Model file for the job. Use its own axes, mm. A direction names the side the tool comes from. Round coordinates to 2 decimals unless told otherwise and drop trailing zeros. Order: outer loops, then holes, each group sorted by start corner. A loop starts at its lowest first (then second) coordinate and runs counter-clockwise, first axis right, second up. Notation, with made-up numbers: (41, 84) - (80, 84) arc R35 cw to (80, 118) - close; hole circle Ø9 at (31, 27.25). An arc over 180 degrees is marked (long way). Answer as CSV lines item,"result". Start each with the question number.
1. Wall check: line 1 along Z through (x, y) = (-33, 35); line 2 along Y through (x, z) = (-4.5, 33.5); line 3 along Z through (x, y) = (-7, 17.5). Give the ranges that are in metal, low to high. Write a range as [from, to].
2. Band-saw the part on D-D on x = -34. List the corners of the cut face in (y, z).
3. Pin check, flat tips, straight feed: pin 1 Ø1.5 at (x, y) = (-9, 22) entering from +Z; pin 2 Ø2.5 at (x, y) = (-34.25, 9.37) entering from -Z; pin 3 Ø5 at (x, y) = (-3.71, 9.37) entering from -Z; pin 4 Ø2.5 at (x, y) = (-34.25, 39.9) entering from +Z. Stop position of each tip, or through.
4. 3-axis set-ups, long thin cutter, end or side, ignore diameter. For faces 1 (the face through (-35.465, 25.364, 33.504)), 2 (the face through (-39.981, 25, 17)), 3 (the face through (-34, 40, 5)): which of +Z, -Z, +X, -X, +Y, -Y reach the whole face in a straight line?
5. Pull direction Y, two halves, no side cores. Call faces 4 (the face through (-4, 40, 5)), 5 (the face through (-22, 27, 35.75)), 6 (the face through (-37.45, 43.17, 16.64)): released by +Y, released by -Y, zero draft, split by the parting line, or undercut.
6. Band-saw the part on B-B on x = -12.5. List the corners of the cut face in (y, z), then the cut area to 3 significant figures.
7. Band-saw the part on C-C on y = 37. List the corners of the cut face in (x, z), then the cut area to 3 significant figures.
8. Band-saw the part on A-A on z = 6. List the corners of the cut face in (x, y).
```python
from build123d import *

# Parameters (mm, degrees)
BOSS_EXTRUDE1_DEPTH = 33.75
SKETCH2_R           = 16.5
CUT_EXTRUDE1_DEPTH  = 0.5
SKETCH3_R           = 11
BOSS_EXTRUDE2_DEPTH = 2.5
SKETCH4_R           = 3.5
CUT_EXTRUDE2_DEPTH  = 5
BOSS_EXTRUDE3_DEPTH = 27
SKETCH6_R           = 1.5
CUT_EXTRUDE3_DEPTH  = 5


with BuildPart() as part:
    # Sketch1 → Boss-Extrude1 (new body)
    with BuildSketch(Plane.XY):
        Polygon((-34.980846502, 45.63851346), (-39.980846502, 40.63851346), (-39.980846502, 8.63851346), (-34.980846502, 3.63851346), (-2.980846502, 3.63851346), (2.019153498, 8.63851346), (2.019153498, 40.63851346), (-2.980846502, 45.63851346), align=None)
    extrude(amount=BOSS_EXTRUDE1_DEPTH)

    # Sketch2 → Cut-Extrude1 (cut)
    with BuildSketch(Plane.XY.offset(33.75)):
        with Locations((-18.980846502, 24.63851346)):
            Circle(SKETCH2_R)
    extrude(amount=-CUT_EXTRUDE1_DEPTH, mode=Mode.SUBTRACT)

    # Sketch3 → Boss-Extrude2 (add)
    with BuildSketch(Plane.XY.offset(33.25)):
        with Locations((-18.980846502, 24.63851346)):
            Circle(SKETCH3_R)
    extrude(amount=BOSS_EXTRUDE2_DEPTH)

    # Sketch4 → Cut-Extrude2 (cut)
    with BuildSketch(Plane.XY.offset(35.75)):
        with Locations((-18.980846502, 24.63851346)):
            Circle(SKETCH4_R)
    extrude(amount=-CUT_EXTRUDE2_DEPTH, mode=Mode.SUBTRACT)

    # Sketch5 → Boss-Extrude3 (add)
    with BuildSketch(Plane.XY.offset(30.75)):
        with BuildLine():
            Line((-20.480846502, 26.63851346), (-17.480846502, 26.63851346))
            ThreePointArc((-17.480846502, 26.63851346), (-18.980846502, 22.13851346), (-20.480846502, 26.63851346))
        make_face()
    extrude(amount=BOSS_EXTRUDE3_DEPTH)

    # Sketch6 → Cut-Extrude3 (cut)
    with BuildSketch(Plane.XY.offset(33.75)):
        with Locations((-34.247281908, 39.904948866)):
            Circle(SKETCH6_R)
        with Locations((-3.714411096, 39.904948866)):
            Circle(SKETCH6_R)
        with Locations((-3.714411096, 9.372078054)):
            Circle(SKETCH6_R)
        with Locations((-34.247281908, 9.372078054)):
            Circle(SKETCH6_R)
    cut_extrude3 = extrude(amount=-CUT_EXTRUDE3_DEPTH, mode=Mode.SUBTRACT)

    # Mirror1: Cut-Extrude3 across plane
    add(cut_extrude3.mirror(Plane(origin=(0, 0, 16.875), x_dir=(1, 0, 0), z_dir=(0, 0, -1))), mode=Mode.SUBTRACT)


solid = part.part
```
Reply:
1,line 1,"z = [0, 33.75]"
1,line 2,"y = [3.64, 8.09], [10.65, 16.73], [32.55, 38.63], [41.18, 45.64]"
1,line 3,"z = [0, 33.25]"
2,outline,"(3.64, 0) - (7.89, 0) - (7.89, 5) - (10.85, 5) - (10.85, 0) - (38.43, 0) - (38.43, 5) - (41.38, 5) - (41.38, 0) - (45.64, 0) - (45.64, 33.75) - (41.38, 33.75) - (41.38, 28.75) - (38.43, 28.75) - (38.43, 33.75) - (31.47, 33.75) - (31.47, 33.25) - (17.81, 33.25) - (17.81, 33.75) - (10.85, 33.75) - (10.85, 28.75) - (7.89, 28.75) - (7.89, 33.75) - (3.64, 33.75) - close"
3,pin 1,"stops at z = 35.75"
3,pin 2,"stops at z = 5"
3,pin 3,"stops at z = 0"
3,pin 4,"stops at z = 28.75"
4,face 1,"+Z"
4,face 2,"+Z, -Z, -X, +Y, -Y"
4,face 3,"-Z"
5,face 4,"undercut"
5,face 5,"zero draft"
5,face 6,"released by +Y"
6,outline,"(3.64, 0) - (45.64, 0) - (45.64, 33.75) - (39.81, 33.75) - (39.81, 33.25) - (33.53, 33.25) - (33.53, 35.75) - (15.75, 35.75) - (15.75, 33.25) - (9.46, 33.25) - (9.46, 33.75) - (3.64, 33.75) - close"
6,area,"1,450 mm2"
7,outline,"(-39.98, 0) - (2.02, 0) - (2.02, 33.75) - (-8.05, 33.75) - (-8.05, 33.25) - (-29.91, 33.25) - (-29.91, 33.75) - (-39.98, 33.75) - close"
7,area,"1,410 mm2"
8,outline,"(-39.98, 8.64) - (-34.98, 3.64) - (-2.98, 3.64) - (2.02, 8.64) - (2.02, 40.64) - (-2.98, 45.64) - (-34.98, 45.64) - (-39.98, 40.64) - close"
